Autodesk Inventor part; units mm, degrees
ref_plane "XZ Plane" through (0, 0, 0) normal (0, 1, 0) x (-1, 0, 0)
ref_plane "XY Plane" through (0, 0, 0) normal (0, 0, 1) x (1, 0, 0)
sketch "Sketch1" plane through (0, 0, 0) normal (0, 0, 1) x (1, 0, 0)
  circle A0 centre (0, 0) radius 3.25
  circle A1 centre (0, 0) radius 11.75
  dimension "d0" = 6.5
  dimension "d1" = 23.5
extrude "Extrusion1" add sketch "Sketch1" along normal blind 3
sketch "Sketch2" plane through (0, 0, 3) normal (0, 0, 1) x (1, 0, 0)
  circle A0 centre (0, 0) radius 3.25
  circle A1 centre (0, 0) radius 4
  dimension "d4" = 8
extrude "Extrusion2" add sketch "Sketch2" along normal blind 15
sketch "Sketch3" plane through (0, 0, 18) normal (0, 0, 1) x (1, 0, 0)
  circle A0 centre (0, 0) radius 3.25
  circle A1 centre (0, 0) radius 6
  dimension "d7" = 12
extrude "Extrusion3" add sketch "Sketch3" along normal blind 2
sketch "Sketch4" plane through (0, 0, 20) normal (0, 0, 1) x (1, 0, 0)
  circle A0 centre (0, 0) radius 3.25
  line L0 (6, 6) -> (-6, 6)
  line L1 (-6, 6) -> (-6, -6)
  line L2 (-6, -6) -> (6, -6)
  line L3 (6, -6) -> (6, 6)
  line L4 (6, 6) -> (-6, -6) construction
  line L5 (-6, 6) -> (6, -6) construction
  circle A1 centre (0, 0) radius 6
extrude "Extrusion4" add sketch "Sketch4" along normal blind 10
sketch "Sketch5" plane through (0, 0, 30) normal (0, 0, 1) x (1, 0, 0)
  circle A0 centre (0, 0) radius 3.25
  circle A1 centre (0, 0) radius 6
extrude "Extrusion5" add sketch "Sketch5" along normal blind 2
sketch "Sketch6" plane through (0, 0, 32) normal (0, 0, 1) x (1, 0, 0)
  circle A0 centre (0, 0) radius 3.25
  circle A1 centre (0, 0) radius 4
extrude "Extrusion6" add sketch "Sketch6" along normal blind 45
sketch "Sketch7" plane through (0, 0, 77) normal (0, 0, 1) x (1, 0, 0)
  circle A0 centre (0, 0) radius 3.25
  circle A1 centre (0, 0) radius 5
  dimension "d16" = 10
extrude "Extrusion7" add sketch "Sketch7" along normal blind 6
sketch "Sketch8" plane through (0, 0, 83) normal (0, 0, 1) x (1, 0, 0)
  circle A0 centre (0, 0) radius 3.25
  circle A1 centre (0, 0) radius 4
extrude "Extrusion8" add sketch "Sketch8" along normal blind 10
sketch "Sketch9" plane through (0, 0, 93) normal (0, 0, 1) x (1, 0, 0)
  circle A0 centre (0, 0) radius 3.25
  circle A1 centre (0, 0) radius 6
extrude "Extrusion9" add sketch "Sketch9" along normal blind 2
sketch "Sketch10" plane through (0, 0, 95) normal (0, 0, 1) x (1, 0, 0)
  circle A0 centre (0, 0) radius 3.25
  line L0 (6, -6) -> (6, 0)
  line L1 (0, -6) -> (6, -6)
  line L2 (-6, -6) -> (0, -6)
  line L3 (-6, 0) -> (-6, -6)
  line L4 (-6, 6) -> (-6, 0)
  line L5 (0, 6) -> (-6, 6)
  line L6 (6, 6) -> (0, 6)
  line L7 (6, 0) -> (6, 6)
extrude "Extrusion10" add sketch "Sketch10" along normal blind 10
sketch "Sketch11" plane through (0, 0, 105) normal (0, 0, 1) x (1, 0, 0)
  circle A0 centre (0, 0) radius 3.25
  circle A1 centre (0, 0) radius 6
extrude "Extrusion11" add sketch "Sketch11" along normal blind 2
ref_plane "Work Plane1" through (5, 0, 77) normal (1, 0, 0) x (0, 1, 0)
sketch "Sketch12" plane through (5, 0, 77) normal (1, 0, 0) x (0, 1, 0)
  line L0 (5, 0) -> (5, 6)
  line L1 (5, 0) -> (-5, 0)
  circle A0 centre (0, 3) radius 1
  point P0 (0, -77)
  point P1 (5, 3)
  point P2 (0, 0)
  dimension "d27" = 2
extrude "Extrusion12" add sketch "Sketch12" along normal blind 5 and the other way blind 0.5
pattern_circular "Circular Pattern1" count 8 over 360 about axis through (0, 0, 32) along (0, 0, 1) of "Extrusion12"
properties part number "039"
Part model, mm, in its own coordinate system. A direction names the side the tool comes from. Coordinates: 2 decimals unless noted, no trailing zeros.
Item 1: Mould opens along Z. For faces 1 (the face through (-7, 0, 79)), 2 (the face through (0, -6, 100)), 3 (the face through (-5, -5, 105)), 4 (the face through (-0.867, 3.905, 10.395)) say: released by +Z, released by -Z, zero draft, split by the parting line, or undercut.
Item 2: Which spindle directions (+Z, -Z, +X, -X, +Y, -Y) get a long thin tool onto all of the face, cutting with end or side? Do faces 5 (the face through (5, -5, 95)), 6 (the face through (-5, 5, 30)), 7 (the face through (-10, 0, 80)), 8 (the face through (6, 0, 100)). Say none if no direction does.
Item 3: Probe line 1 (Y direction, x = 0, z = 39.5); line 2 (Y direction, x = 0, z = 25); line 3 (X direction, y = -1.5, z = 64.5). List the from-to ranges inside material, lowest first.
Item 4: Pin check, flat tips, straight feed: pin 1 (11 mm diameter, centred on x = 1, z = 26, fed in from -Y); pin 2 (3 mm diameter, centred on x = 1.5, z = 23, fed in from +Y); pin 3 (12 mm diameter, centred on y = 8.5, z = 86, fed in from +X). Stop position of each tip, or through.
Results found:
1. face 1: undercut
1. face 2: zero draft
1. face 3: released by +Z
1. face 4: undercut
2. face 5: +X, -Y
2. face 6: -X, +Y
2. face 7: +Z, -X, +Y, -Y
2. face 8: +Z, +X, +Y, -Y
3. line 1: y = -4 to -3.25, 3.25 to 4
3. line 2: y = -6 to -3.25, 3.25 to 6
3. line 3: x = -3.71 to -2.88, 2.88 to 3.71
4. pin 1: stops at y = -6
4. pin 2: stops at y = 6
4. pin 3: stops at x = 7.73
